Autodesk Inventor part; units mm, degrees
ref_plane "YZ Plane" through (0, 0, 0) normal (1, 0, 0) x (0, 1, 0)
ref_plane "XZ Plane" through (0, 0, 0) normal (0, 1, 0) x (-1, 0, 0)
ref_plane "XY Plane" through (0, 0, 0) normal (0, 0, 1) x (1, 0, 0)
sketch "Sketch1" plane through (0, 0, 0) normal (0, 0, 1) x (1, 0, 0)
  line L0 (-6, 5) -> (6, 5)
  line L1 (6, 5) -> (6, 0)
  line L2 (6, 0) -> (-6, 0)
  line L3 (-6, 0) -> (-6, 5)
  line L4 (-6, 5) -> (6, 0) construction
  line L5 (6, 5) -> (-6, 0) construction
  line L6 (-13.5, 10) -> (13.5, 10)
  line L7 (13.5, 10) -> (13.5, 0)
  line L8 (13.5, 0) -> (-13.5, 0)
  line L9 (-13.5, 0) -> (-13.5, 10)
  line L10 (-13.5, 10) -> (13.5, 0) construction
  line L11 (13.5, 10) -> (-13.5, 0) construction
  point P0 (0, 0)
  point P1 (0, 2.5)
  point P2 (0, 0)
  point P3 (0, 5)
  point P4 (6, 0)
  point P5 (-6, 0)
  dimension "d0" = 12
  dimension "d1" = 5
  dimension "d2" = 27
  dimension "d3" = 10
extrude "Extrusion1" add sketch "Sketch1" along normal mid plane 34.7 contours L3 L8 L9 L6 L7 L1 L0
sketch "Sketch2" plane through (-13.5, 10, 17.35) normal (0, 1, 0) x (1, 0, 0)
  line L0 (23.5, 9.85) -> (3.5, 9.85) construction
  line L1 (3.5, 9.85) -> (3.5, 24.85) construction
  line L2 (3.5, 24.85) -> (23.5, 24.85) construction
  line L3 (23.5, 24.85) -> (23.5, 9.85) construction
  line L4 (23.5, 9.85) -> (3.5, 24.85) construction
  line L5 (3.5, 9.85) -> (23.5, 24.85) construction
  point P0 (13.5, 17.35)
  dimension "d6" = 20
  dimension "d7" = 15
hole "Hole1" at (-10, 10, 7.5) at (10, 10, 7.5) at (10, 10, -7.5) at (-10, 10, -7.5) direction (0, -1, 0) diameter 2.459 depth 4
fillet "Fillet1" radius 1 4 edges at (13.5, 10, 0) (-13.5, 10, 0) (13.5, 0, 0) (-13.5, 0, 0)
properties part number "MGN12C Cart" material "Steel, Carbon"
Input: part model. Units: mm. Frame: model coordinates. A direction names the side the tool comes from. Coordinates: 2 decimals unless noted, no trailing zeros. Loops run counter-clockwise (first coordinate to the right, second up) from the corner with the lowest first, then second, coordinate; pieces in that order, holes last. Notation, with made-up numbers: (42.5, 14.5) -> (56.5, 14.5) arc R24 ccw to (56.5, 30.5) -> close; hole circle Ø9 at (66.25, 88.25). An arc over 180 degrees is marked (long way). One line per item, written item: value.
(1) Cut plane A-A (z = 7.5). Output: boundary loops of the cut face in (x, y), then the cut area to 3 significant figures.
Answer below:
outline: (-13.5, 1) arc R1 ccw to (-12.5, 0) -> (-6, 0) -> (-6, 5) -> (6, 5) -> (6, 0) -> (12.5, 0) arc R1 ccw to (13.5, 1) -> (13.5, 9) arc R1 ccw to (12.5, 10) -> (11.23, 10) -> (11.23, 6) -> (8.77, 6) -> (8.77, 10) -> (-8.77, 10) -> (-8.77, 6) -> (-11.23, 6) -> (-11.23, 10) -> (-12.5, 10) arc R1 ccw to (-13.5, 9) -> close
area: 189 mm2
(2) Ray query, line 1 along X through (y, z) = (8.25, -7.5); line 2 along Z through (x, y) = (-10, 8.5); line 3 along X through (y, z) = (2.25, -2). Return the intervals inside material, ascending.
Answer below:
line 1: x = -13.5 to -11.23, -8.77 to 8.77, 11.23 to 13.5
line 2: z = -17.35 to -8.73, -6.27 to 6.27, 8.73 to 17.35
line 3: x = -13.5 to -6, 6 to 13.5
(3) Set-up query: faces 5 (the face through (13.5, 5, 0)), 6 (the face through (6, 3, 0)), 7 (the face through (11.09, 7.97, -6.93)). Return all of +Z, -Z, +X, -X, +Y, -Y with unobstructed straight access to the full face (end or side cutting, diameter ignored); none if empty.
Answer below:
face 5: +Z, -Z, +X, +Y, -Y
face 6: +Z, -Z, -Y
face 7: +Y
(4) Cut plane C-C (z = 13). Output: boundary loops of the cut face in (x, y), then the cut area to 3 significant figures.
Answer below:
outline: (-13.5, 1) arc R1 ccw to (-12.5, 0) -> (-6, 0) -> (-6, 5) -> (6, 5) -> (6, 0) -> (12.5, 0) arc R1 ccw to (13.5, 1) -> (13.5, 9) arc R1 ccw to (12.5, 10) -> (-12.5, 10) arc R1 ccw to (-13.5, 9) -> close
area: 209 mm2
(5) Pin query (flat end, axial travel): pin 1 Ø6 at (x, z) = (1.5, 2.5) entering from -Y; pin 2 Ø1.5 at (x, z) = (10, -7.5) entering from +Y. Return the tip coordinate at first contact, or that it passes through.
Answer below:
pin 1: stops at y = 5
pin 2: stops at y = 6
(6) Cut plane D-D (x = 1.5). Output: boundary loops of the cut face in (y, z), then the cut area to 4 significant figures.
Answer below:
outline: (5, -17.35) -> (10, -17.35) -> (10, 17.35) -> (5, 17.35) -> close
area: 173.5 mm2
(7) Draft query along X for faces 1 (the face through (10, 6, 7)), 2 (the face through (0, 5, 0)), 3 (the face through (-13.5, 5, 0)), 4 (the face through (9, 0, 0)). Return one class per face: pulls with the +X half, pulls with the -X half, needs draft (parallel to the pull), parting line crosses it, or undercut.
Answer below:
face 1: undercut
face 2: undercut
face 3: pulls with the -X half
face 4: needs draft
(8) Cut plane B-B (x = 10). Output: boundary loops of the cut face in (y, z).
Answer below:
outline: (0, -17.35) -> (10, -17.35) -> (10, -8.73) -> (6, -8.73) -> (6, -6.27) -> (10, -6.27) -> (10, 6.27) -> (6, 6.27) -> (6, 8.73) -> (10, 8.73) -> (10, 17.35) -> (0, 17.35) -> close
